Check sheet for the modelled part. Datum: model origin and axes. Units: mm. A direction names the side the tool comes from. Round coordinates to 2 decimals unless told otherwise and drop trailing zeros. Write each loop counter-clockwise with the first axis right and the second up, starting at its lowest first coordinate (ties: lowest second). Pieces come first, ordered by that corner, then holes.
Item 1: Tool access check on faces 1 (the cylindrical face through (73.95, 6.26, 6.32)), 2 (the flat face through (-22, 8.9, -33)). Record the directions out of +Z, -Z, +X, -X, +Y, -Y that give a thin tool (end or side, any length) a straight path to the whole face; none if there is none.
Item 2: Go/stop test with flat-tipped pins: pin 1 Ø3 at (x, y) = (26, 7) entering from +Z; pin 2 Ø6.5 at (x, y) = (64, 5.5) entering from +Z; pin 3 Ø4 at (x, y) = (-56, 8.5) entering from -Z. Record where each tip stops, or that it passes through.
Item 3: Material ranges on line 1 (X direction, y = 7.75, z = 12); line 2 (Z direction, x = 16, y = 11); line 3 (X direction, y = 3.25, z = 62.5), recorded low to high.
Item 4: Cross-section at B-B on y = 3.75. Count the separate pieces of the cut face and the enclosed holes in it, plus the area to 3 significant figures.
Item 5: Cross-section at A-A on z = 0. Enter the section's corners in (x, y), plus the area to 3 significant figures.
from build123d import *

# Parameters (mm, degrees)
F_12_0_189_DIAMETER_HOLE1_D = 4.8006
CIRPATTERN3_COUNT           = 6
CUT_EXTRUDE1_DEPTH          = 13.7
FILLET1_R                   = 4
CIRPATTERN4_COUNT           = 6
FILLET1_OF_CIRPATTERN4_R    = 4
CHAMFER1_SIZE               = 1
CHAMFER2_SIZE               = 1


with BuildPart() as part:
    # Sketch2 → Revolve1 (revolve)
    with BuildSketch(Plane(origin=(0, 0, 0), x_dir=(0, 0, -1), z_dir=(1, 0, 0))):
        Polygon((-39.2125, 0), (-80.55, 0), (-80.55, 12.7), (-49.2125, 12.7), (-49.2125, 8.9), (-39.2125, 8.9), align=None)
    revolve(axis=Axis((0, -0.635, 0), (0, 1, 0)))

    # #12 (0.189) Diameter Hole1 (through all)
    with Locations(Plane(origin=(0, 12.7, 0), x_dir=(1, 0, 0), z_dir=(0, 1, 0))):
        with Locations((-35, 60.621778)):
            f_12_0_189_diameter_hole1 = Hole(F_12_0_189_DIAMETER_HOLE1_D / 2)

    # CirPattern3: #12 (0.189) Diameter Hole1 ×6 about axis
    cirpattern3_axis = Axis((0, 0, 0), (0, 1, 0))
    for i in range(1, CIRPATTERN3_COUNT):
        add(f_12_0_189_diameter_hole1.rotate(cirpattern3_axis, i * 360 / CIRPATTERN3_COUNT), mode=Mode.SUBTRACT)

    # Sketch8 → Cut-Extrude1 (cut, through all)
    with BuildSketch(Plane(origin=(0, 12.7, 0), x_dir=(1, 0, 0), z_dir=(0, 1, 0))):
        with BuildLine():
            Line((-33.362056, 67.784775), (-22.66059, 49.249293))
            ThreePointArc((-22.66059, 49.249293), (0, 54.2125), (22.66059, 49.249293))
            Line((22.66059, 49.249293), (33.362056, 67.784775))
            ThreePointArc((33.362056, 67.784775), (0, 75.55), (-33.362056, 67.784775))
        make_face()
    cut_extrude1 = extrude(amount=-CUT_EXTRUDE1_DEPTH, mode=Mode.SUBTRACT)

    # Fillet1
    fillet1_edges = [part.edges().sort_by_distance(p)[0] for p in [
        (22.66059, 6.35, -49.249293),
        (-22.66059, 6.35, -49.249293),
        (-33.362056, 6.35, -67.784775),
        (33.362056, 6.35, -67.784775),
    ]]
    fillet(fillet1_edges, radius=FILLET1_R)

    # CirPattern4: Cut-Extrude1 ×6 about axis
    cirpattern4_axis = Axis((0, 0, 0), (0, 1, 0))
    for i in range(1, CIRPATTERN4_COUNT):
        add(cut_extrude1.rotate(cirpattern4_axis, i * 360 / CIRPATTERN4_COUNT), mode=Mode.SUBTRACT)

    # Fillet1 of CirPattern4
    fillet1_of_cirpattern4_edges = [part.edges().sort_by_distance(p)[0] for p in [
        (-31.320844, 6.35, -44.249293),
        (-53.981433, 6.35, -5),
        (-75.384365, 6.35, -5),
        (-42.02231, 6.35, -62.784775),
        (-53.981433, 6.35, 5),
        (-31.320844, 6.35, 44.249293),
        (-42.02231, 6.35, 62.784775),
        (-75.384365, 6.35, 5),
        (-22.66059, 6.35, 49.249293),
        (22.66059, 6.35, 49.249293),
        (33.362056, 6.35, 67.784775),
        (-33.362056, 6.35, 67.784775),
        (31.320844, 6.35, 44.249293),
        (53.981433, 6.35, 5),
        (75.384365, 6.35, 5),
        (42.02231, 6.35, 62.784775),
        (53.981433, 6.35, -5),
        (31.320844, 6.35, -44.249293),
        (42.02231, 6.35, -62.784775),
        (75.384365, 6.35, -5),
    ]]
    fillet(fillet1_of_cirpattern4_edges, radius=FILLET1_OF_CIRPATTERN4_R)

    # Chamfer1
    chamfer1_edges = [part.edges().sort_by_distance(p)[0] for p in [
        (0, 12.7, -49.2125),
    ]]
    chamfer(chamfer1_edges, length=CHAMFER1_SIZE)

    # Chamfer2
    chamfer2_edges = [part.edges().sort_by_distance(p)[0] for p in [
        (0, 0, -80.55),
    ]]
    chamfer(chamfer2_edges, length=CHAMFER2_SIZE)


solid = part.part
Response values:
1. face 1: +Y, -Y
1. face 2: +Y
2. pin 1: stops at z = 76.73
2. pin 2: stops at z = 52.89
2. pin 3: stops at z = -59.77
3. line 1: x = -79.65 to -74.59, -52.87 to -37.33, 37.33 to 52.87, 74.59 to 79.65
3. line 2: z = -78.94 to -73.84, -51.8 to -46.54, 46.54 to 51.8, 73.84 to 78.94
3. line 3: x = -50.81 to -36.49, -33.51 to -30.31, 30.31 to 33.51, 36.49 to 50.81
4. separate pieces: 1
4. enclosed holes: 13
4. area: 8,110 mm2
5. outline: (-80.55, 1) - (-79.55, 0) - (-72.4, 0) - (-72.4, 12.7) - (-80.55, 12.7) - close; (-67.6, 0) - (-39.21, 0) - (-39.21, 8.9) - (-49.21, 8.9) - (-49.21, 11.7) - (-50.21, 12.7) - (-67.6, 12.7) - close; (39.21, 0) - (67.6, 0) - (67.6, 12.7) - (50.21, 12.7) - (49.21, 11.7) - (49.21, 8.9) - (39.21, 8.9) - close; (72.4, 0) - (79.55, 0) - (80.55, 1) - (80.55, 12.7) - (72.4, 12.7) - close
5. area: 850 mm2
